Read the model definition and answer for the solid it produces. Units are mm, in the model's axes. Face numbers are marked on the shaded views. Coordinates: 2 decimals unless noted, no trailing zeros. Loops run counter-clockwise (first coordinate to the right, second up) from the corner with the lowest first, then second, coordinate; pieces in that order, holes last. Notation, with made-up numbers: (-33, 52.5) - (-27, 52.5) arc R20 ccw to (-27, 82.5) - close; hole circle Ø7 at (54.25, 52). An arc over 180 degrees is marked (long way). Use one line per item in the form item = value.
from build123d import *

# Parameters (mm, degrees)
SKETCH_1_W          = 56
SKETCH_1_H          = 16
EXTRUDE_1_DEPTH     = 1.3
EXTRUDE_2_DEPTH     = 1.3
FILLET_1_R          = 2
FILLET_2_R          = 0.5
CHAMFER_1_SIZE      = 2
CHAMFER_1_SIZE_2    = 2.383507185
CHAMFER_2_SIZE      = 2.383507185
CHAMFER_2_SIZE_2    = 2
SKETCH_3_W          = 1.5
SKETCH_3_H          = 8
EXTRUDE_3_DEPTH     = 1.1
CHAMFER_3_SIZE      = 1
SKETCH_4_W          = 28.445563285
SKETCH_4_H          = 1.4
EXTRUDE_4_DEPTH     = 2.5
FILLET_3_R          = 1.4
CUT_EXTRUDE_1_REACH = 33.803
SKETCH_6_W          = 8
SKETCH_6_H          = 10
FILLET_4_R          = 1.4


# Some blends are built 0.0001 mm under size
with BuildPart() as part:
    # 草图1 → 凸台-拉伸1 (new body)
    with BuildSketch(Plane.XY):
        Rectangle(SKETCH_1_W, SKETCH_1_H)
    extrude(amount=EXTRUDE_1_DEPTH)

    # 草图2 → 凸台-拉伸2 (add)
    with BuildSketch(Plane.XY.offset(1.3)):
        Polygon((28, 8), (30.2, 8), (30.2, 0), (31, 0), (31, -2), (29, -2), (29, 6), (28, 6), align=None)
        Polygon((-28, 8), (-30.2, 8), (-30.2, 0), (-31, 0), (-31, -2), (-29, -2), (-29, 6), (-28, 6), align=None)
    extrude(amount=-EXTRUDE_2_DEPTH)

    # 圆角1
    fillet_1_edges = [part.edges().sort_by_distance(p)[0] for p in [
        (-30.2, 8, 0.65),
        (30.2, 8, 0.65),
        (28, -8, 0.65),
        (-28, -8, 0.65),
    ]]
    fillet(fillet_1_edges, radius=FILLET_1_R)

    # 圆角2
    fillet_2_edges = [part.edges().sort_by_distance(p)[0] for p in [
        (28, 6, 0.65),
        (29, 6, 0.65),
        (-28, 6, 0.65),
        (-29, 6, 0.65),
    ]]
    fillet(fillet_2_edges, radius=FILLET_2_R - 0.0001)  # a hair under: the kernel refuses the full size

    # 倒角1
    # the kernel refuses this chamfer: 2.383507185, 2 mm, written as the material it takes off along each edge
    with BuildSketch(Plane(origin=(31, -2, 7.443265966), x_dir=(-0.9993728857116145, -0.03540953691366299, 0), z_dir=(0, 0, -1))) as chamfer_1_piece_1:
        Polygon((CHAMFER_1_SIZE * 0.999372885712, CHAMFER_1_SIZE * 0.0354095369137), (-CHAMFER_1_SIZE_2 * 0.0354095369165, CHAMFER_1_SIZE_2 * 0.999372885791), (0, 0), align=None)
    extrude(amount=13.586531933, mode=Mode.SUBTRACT)

    # 倒角2
    # the kernel refuses this chamfer: 2.383507185, 2 mm, written as the material it takes off along each edge
    with BuildSketch(Plane(origin=(-31, -2, 7.443265966), x_dir=(-0.024939322090233737, 0.9996889667359941, 0), z_dir=(0, 0, -1))) as chamfer_2_piece_1:
        Polygon((CHAMFER_2_SIZE * 0.999688966815, CHAMFER_2_SIZE * 0.0249393220922), (-CHAMFER_2_SIZE_2 * 0.0249393220902, CHAMFER_2_SIZE_2 * 0.999688966736), (0, 0), align=None)
    extrude(amount=13.586531933, mode=Mode.SUBTRACT)

    # 草图3 → 凸台-拉伸3 (add)
    with BuildSketch(Plane.XY.offset(1.3)):
        with Locations((-13.15891381, -1.11681071)):
            Rectangle(SKETCH_3_W, SKETCH_3_H)
        with Locations((13.84108619, -1.11681071)):
            Rectangle(SKETCH_3_W, SKETCH_3_H)
    extrude(amount=EXTRUDE_3_DEPTH)

    # 倒角3
    chamfer_3_edges = [part.edges().sort_by_distance(p)[0] for p in [
        (-13.15891381, -5.11681071, 2.4),
        (-13.15891381, 2.88318929, 2.4),
        (13.84108619, -5.11681071, 2.4),
        (13.84108619, 2.88318929, 2.4),
    ]]
    chamfer(chamfer_3_edges, length=CHAMFER_3_SIZE)

    # 草图4 → 凸台-拉伸4 (add)
    with BuildSketch(Plane.XY.offset(1.3)):
        with Locations((0.313867832, -1.81681071)):
            Rectangle(SKETCH_4_W, SKETCH_4_H)
    extrude(amount=EXTRUDE_4_DEPTH)

    # 圆角3
    fillet_3_edges = [part.edges().sort_by_distance(p)[0] for p in [
        (14.536649475, -1.81681071, 3.8),
        (-13.90891381, -1.81681071, 3.8),
    ]]
    fillet(fillet_3_edges, radius=FILLET_3_R - 0.0001)  # a hair under: the kernel refuses the full size

    # 草图6 → 切除-拉伸1 (cut, up to next)
    with BuildSketch(Plane.XY.offset(1.3), mode=Mode.PRIVATE) as cut_extrude_1_sk1:
        with Locations((-21, 0)):
            Rectangle(SKETCH_6_W, SKETCH_6_H)
    cut_extrude_1_tool1 = extrude(cut_extrude_1_sk1.sketch, amount=-CUT_EXTRUDE_1_REACH, mode=Mode.PRIVATE) & part.part
    # 草图6 → 切除-拉伸1 (cut, up to next)
    with BuildSketch(Plane.XY.offset(1.3), mode=Mode.PRIVATE) as cut_extrude_1_sk2:
        with Locations((21, 0)):
            Rectangle(SKETCH_6_W, SKETCH_6_H)
    cut_extrude_1_tool2 = extrude(cut_extrude_1_sk2.sketch, amount=-CUT_EXTRUDE_1_REACH, mode=Mode.PRIVATE) & part.part
    add(cut_extrude_1_tool1.solids().sort_by_distance((-21, 0, 1.3))[0], mode=Mode.SUBTRACT)
    add(cut_extrude_1_tool2.solids().sort_by_distance((21, 0, 1.3))[0], mode=Mode.SUBTRACT)

    # 圆角4
    fillet_4_edges = [part.edges().sort_by_distance(p)[0] for p in [
        (-17, 5, 0.65),
        (-17, -5, 0.65),
        (-25, -5, 0.65),
        (-25, 5, 0.65),
        (25, 5, 0.65),
        (25, -5, 0.65),
        (17, -5, 0.65),
        (17, 5, 0.65),
    ]]
    fillet(fillet_4_edges, radius=FILLET_4_R)


solid = part.part
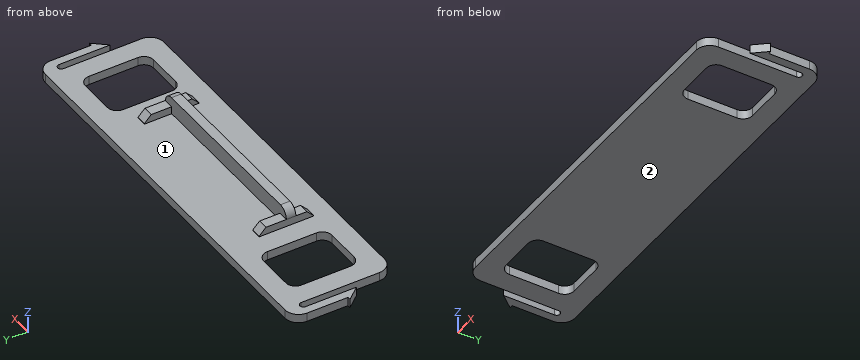
Item 1: The part is cut by section B-B on x = -20. Give the vertices of the cut face in (y, z).
Results below:
outline = (-8, 0) - (-5, 0) - (-5, 1.3) - (-8, 1.3) - close; (5, 0) - (8, 0) - (8, 1.3) - (5, 1.3) - close
Item 2: The part is cut by section A-A on y = 1. Give the vertices of the cut face in (x, z), plus the area to 3 significant figures.
Results below:
outline = (-30.2, 0) - (-29, 0) - (-29, 1.3) - (-30.2, 1.3) - close; (-28, 0) - (-25, 0) - (-25, 1.3) - (-28, 1.3) - close; (-17, 0) - (17, 0) - (17, 1.3) - (14.59, 1.3) - (14.59, 2.4) - (13.09, 2.4) - (13.09, 1.3) - (-12.41, 1.3) - (-12.41, 2.4) - (-13.91, 2.4) - (-13.91, 1.3) - (-17, 1.3) - close; (25, 0) - (28, 0) - (28, 1.3) - (25, 1.3) - close; (29, 0) - (30.2, 0) - (30.2, 1.3) - (29, 1.3) - close
area = 58.4 mm²
Item 3: The part is cut by section C-C on x = -7. Give the vertices of the cut face in (y, z).
Results below:
outline = (-8, 0) - (8, 0) - (8, 1.3) - (-1.12, 1.3) - (-1.12, 3.8) - (-2.52, 3.8) - (-2.52, 1.3) - (-8, 1.3) - close
Item 4: For a pull along X with two mould halves and no side action, classify the marked faces 1 and 2 as +X half, -X half, draft (parallel to the pull), parting line (faces both ways), or undercut.
Results below:
face_1 = undercut
face_2 = draft
Item 5: The part is cut by section D-D on z = 2.95. Give the vertices of the cut face in (x, y), plus the area to 3 significant figures.
Results below:
outline = (-13.8, -2.52) - (14.42, -2.52) - (14.42, -1.12) - (-13.8, -1.12) - close
area = 39.5 mm²
Item 6: Find the intervals of material crossed by L1, parallel to X at y = 1.25, z = 0.4; L2, parallel to X at y = -2.25, z = 0.5; L3, parallel to X at y = -0.5, z = 1.55, in increasing order.
Results below:
L1 = -30.2 to -29, -28 to -25, -17 to 17, 25 to 28, 29 to 30.2
L2 = -28 to -25, -17 to 17, 25 to 28
L3 = -13.91 to -12.41, 13.09 to 14.59
Item 7: Each of these flat-tipped pins is pushed along its axis until it touches: P1, Ø0.6, axis at y = -0.5, z = 0.5, coming from the +X side; P2, Ø1.5, axis at x = 22.5, z = 1.5, coming from the -Y side; P3, Ø0.9, axis at y = -2, z = 2, coming from the +X side; P4, Ø1, axis at y = 1.5, z = 1, coming from the +X side. Where does it stop, or does it pass through?
Results below:
P1 = 30.51
P2 = -8
P3 = 14.59
P4 = 30.2
